```python
from build123d import *

# Parameters (mm, degrees)
SKETCH1_W           = 80.9625
SKETCH1_H           = 50.8
SKETCH1_R           = 1.5875
BOSS_EXTRUDE1_DEPTH = 1.5875
FILLET1_R           = 4.7625


with BuildPart() as part:
    # Sketch1 → Boss-Extrude1 (new body)
    with BuildSketch(Plane(origin=(0, 0, 0), x_dir=(1, 0, 0), z_dir=(0, 1, 0))):
        with Locations((40.48125, 25.4)):
            Rectangle(SKETCH1_W, SKETCH1_H)
        with Locations((3.96875, 25.4)):
            Circle(SKETCH1_R, mode=Mode.SUBTRACT)
        with Locations((76.99375, 25.4)):
            Circle(SKETCH1_R, mode=Mode.SUBTRACT)
    extrude(amount=BOSS_EXTRUDE1_DEPTH)

    # Fillet1
    fillet1_edges = [part.edges().sort_by_distance(p)[0] for p in [
        (0, 0.79375, -50.8),
        (80.9625, 0.79375, -50.8),
        (80.9625, 0.79375, 0),
        (0, 0.79375, 0),
    ]]
    fillet(fillet1_edges, radius=FILLET1_R)


solid = part.part
```
Work out the finished part from the listing and answer in its coordinate system (mm). Coordinates: 2 decimals unless noted, no trailing zeros. Loops run counter-clockwise (first coordinate to the right, second up) from the corner with the lowest first, then second, coordinate; pieces in that order, holes last. Notation, with made-up numbers: (68.25, -3) - (109.25, -3) arc R31 ccw to (109.25, 21) - close; hole circle Ø5 at (43.5, 87.5). An arc over 180 degrees is marked (long way). Use a Markdown table: item, result.
Item 1: Given pin 1 Ø3 at (x, z) = (3.97, -25.4) entering from +Y; pin 2 Ø6 at (x, z) = (30.5, -20.5) entering from -Y, each flat-ended and moving along its own axis, determine where each tip first touches the part or whether it passes through.
Evaluation:
| item | result |
|---|---|
| pin 1 | passes through |
| pin 2 | stops at y = 0 |
Item 2: Consider probe 1 along X at (y, z) = (0.8, -25.4); probe 2 along Z at (x, y) = (77.5, 0.9). Determine where each line is inside the solid, lowest interval first. Write a range as from..to.
Evaluation:
| item | result |
|---|---|
| probe 1 | x = 0..2.38, 5.56..75.41, 78.58..80.96 |
| probe 2 | z = -50.62..-26.9, -23.9..-0.18 |
Item 3: Find section A-A, the plane z = -25.4. Determine the outline of the cut face in (x, y).
Evaluation:
| item | result |
|---|---|
| outline | (0, 0) - (2.38, 0) - (2.38, 1.59) - (0, 1.59) - close; (5.56, 0) - (75.41, 0) - (75.41, 1.59) - (5.56, 1.59) - close; (78.58, 0) - (80.96, 0) - (80.96, 1.59) - (78.58, 1.59) - close |
Item 4: The mould has two halves that part along Z. Classify faces 1 (the flat face through (40, 1, 0)), 2 (the cylindrical face through (77.847, 0.783, -26.739)), 3 (the cylindrical face through (1.36, 0.8, -49.37)): +Z half, -Z half, draft (parallel to the pull), parting line (faces both ways), or undercut.
Evaluation:
| item | result |
|---|---|
| face 1 | +Z half |
| face 2 | undercut |
| face 3 | -Z half |
